For this review, use the dimensioned drawing (mm, ordinates from the lowest corner) and the shaded views. A direction names the side the tool comes from. Round coordinates to 2 decimals unless told otherwise and drop trailing zeros. Write each loop counter-clockwise with the first axis right and the second up, starting at its lowest first coordinate (ties: lowest second). Pieces come first, ordered by that corner, then holes. Notation, with made-up numbers: (64, 52) -> (70, 52) arc R17 ccw to (70, 71) -> close; hole circle Ø9 at (-20, 23). An arc over 180 degrees is marked (long way). Answer as CSV lines item,"result". Start each with the question number.
Item 1: Take a section at C-C on x = 20. Give the boundary of the cut face in (y, z).
Item 2: For pin 1 Ø5 at (x, y) = (28.5, 27.5) entering from +Z, flat-tipped, find the tip position at first contact; note if it passes through.
Item 3: Take a section at B-B on y = 22.5. Give the boundary of the cut face in (x, z).
Item 4: Take a section at A-A on z = 2. Give the boundary of the cut face in (x, y), then the cut area to 3 significant figures.
Item 5: Machinability: for the marked faces 1, 2 and 3, which of the approach directions +Z, -Z, +X, -X, +Y, -Y give a long, thin tool a straight path to every point of the face, cutting with its end or side? Answer none if there is none.
Item 6: Mouldability with a two-part tool opening along X and no side actions: class the marked faces 4, 5 and 6 as +X half, -X half, draft (parallel to the pull), parting line (faces both ways), or undercut.
Item 7: Wall thickness on probe 1 along X at (y, z) = (22.5, 6); probe 2 along X at (y, z) = (13, 2.75); probe 3 along Z at (x, y) = (20, 5): over which ranges is each line inside the solid? List them lowest first. Write a range as from..to.
Item 8: Take a section at D-D on x = 29. Give the boundary of the cut face in (y, z).
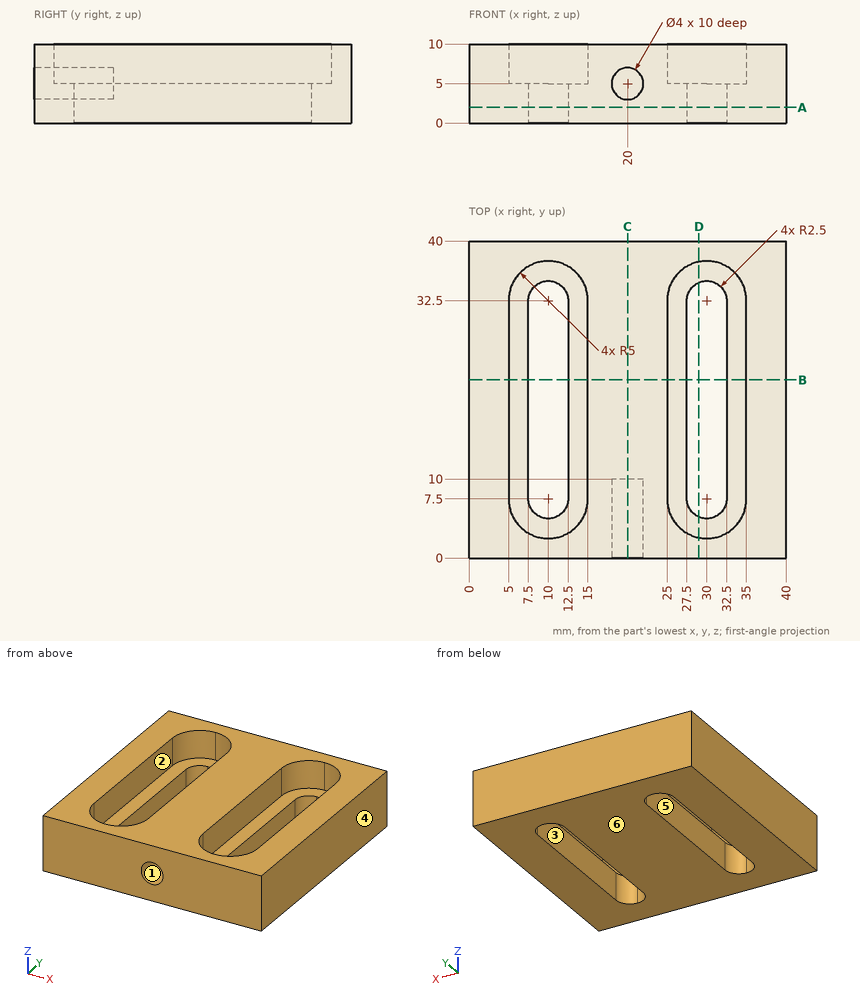
Output values:
1,outline,"(0, 0) -> (40, 0) -> (40, 10) -> (0, 10) -> (0, 7) -> (10, 7) -> (10, 3) -> (0, 3) -> close"
2,pin 1,"stops at z = 5"
3,outline,"(0, 0) -> (7.5, 0) -> (7.5, 5) -> (5, 5) -> (5, 10) -> (0, 10) -> close; (12.5, 0) -> (27.5, 0) -> (27.5, 5) -> (25, 5) -> (25, 10) -> (15, 10) -> (15, 5) -> (12.5, 5) -> close; (32.5, 0) -> (40, 0) -> (40, 10) -> (35, 10) -> (35, 5) -> (32.5, 5) -> close"
4,outline,"(0, 0) -> (40, 0) -> (40, 40) -> (0, 40) -> close; hole (7.5, 7.5) arc R2.5 ccw to (12.5, 7.5) -> (12.5, 32.5) arc R2.5 ccw to (7.5, 32.5) -> close; hole (27.5, 7.5) arc R2.5 ccw to (32.5, 7.5) -> (32.5, 32.5) arc R2.5 ccw to (27.5, 32.5) -> close"
4,area,"1,310 mm^2"
5,face 1,"-Y"
5,face 2,"+Z"
5,face 3,"+Z, -Z"
6,face 4,"+X half"
6,face 5,"undercut"
6,face 6,"draft"
7,probe 1,"x = 0..5, 15..25, 35..40"
7,probe 2,"x = 0..7.5, 12.5..27.5, 32.5..40"
7,probe 3,"z = 0..3, 7..10"
8,outline,"(0, 0) -> (5.21, 0) -> (5.21, 5) -> (2.6, 5) -> (2.6, 10) -> (0, 10) -> close; (34.79, 0) -> (40, 0) -> (40, 10) -> (37.4, 10) -> (37.4, 5) -> (34.79, 5) -> close"
